Autodesk Fusion 360 part; units mm, degrees
sketch "Sketch1" plane through (0, 0, 0) normal (0, 0, 1) x (1, 0, 0)
  line L0 (0, 0) -> (-45, 0)
  line L1 (0, 0) -> (0, 45)
  line L2 (0, 45) -> (-45, 0)
  line L3 (-5, 40) -> (-5, 5)
  line L4 (-5, 5) -> (-40, 5)
  line L5 (-2, 43) -> (0, 43)
  line L6 (-43, 2) -> (-43, 0)
  dimension "d1" = 45
  dimension "d2" = 45
  dimension "d5" = 5
  dimension "d6" = 5
  dimension "d7" = 2
  dimension "d8" = 2
extrude "Extrude2" add sketch "Sketch1" along normal blind 20 contours L0 L1 L2 L3 L4 L5 L6
extrude "Extrude3" add sketch "Sketch1" along normal blind 5 contours L2 L3 L4
Work out the finished part from the listing and answer in its coordinate system (mm). A direction names the side the tool comes from. Coordinates: 2 decimals unless noted, no trailing zeros. Write each loop counter-clockwise with the first axis right and the second up, starting at its lowest first coordinate (ties: lowest second). Pieces come first, ordered by that corner, then holes. Notation, with made-up numbers: M -21.75,32 L -3.75,32 A23 cw -3.75,67 Z; hole C 40.25,88.25 d1. An arc over 180 degrees is marked long. Use one line per item in the form item = value. Start each with the question number.
1. The part is cut by section B-B (x = -37.5). Give the vertices of the cut face in (y, z), plus the area to 4 significant figures.
2. The part is cut by section A-A (y = 39). Give the vertices of the cut face in (x, z).
3. The part is cut by section D-D (z = 15.25). Give the vertices of the cut face in (x, y).
4. Each of these flat-tipped pins is pushed along its axis until it touches: P1, Ø7.5, axis at y = 14.5, z = 10, coming from the -X side; P2, Ø7.5, axis at x = -18, z = 12.5, coming from the +Y side; P3, Ø1.5, axis at x = -12, y = 26, coming from the +Z side. Where does it stop, or does it pass through?
5. The part is cut by section C-C (z = 4.25). Give the vertices of the cut face in (x, y).
6. A tool of negligible diameter and unlimited length cuts with its end or side. For faces 1 (the face through (-15, 15, 5)), 2 (the face through (-22, 23, 3)), from which of +Z, -Z, +X, -X, +Y, -Y can it reach the whole face along a straight path? Write none if from no direction.
7. Straight lines are drawn through the part: probe 1 along X at (y, z) = (35, 8.75); probe 2 along Y at (x, z) = (-21.5, 15.5). For each, find the intervals that lie inside material, in ascending order. Write a range as from..to.
Evaluation:
q1.outline = M 0,0 L 7.5,0 L 7.5,5 L 5,5 L 5,20 L 0,20 Z
q1.area = 112.5 mm^2
q2.outline = M -6,0 L 0,0 L 0,20 L -5,20 L -5,5 L -6,5 Z
q3.outline = M -43,0 L 0,0 L 0,43 L -2,43 L -5,40 L -5,5 L -40,5 L -43,2 Z
q4.P1 = -5
q4.P2 = 5
q4.P3 = 5
q5.outline = M -43,0 L 0,0 L 0,43 L -2,43 L -43,2 Z
q6.face_1 = +Z, -X, +Y
q6.face_2 = +Z, -Z, -X, +Y
q7.probe_1 = -5..0
q7.probe_2 = 0..5
